Check sheet for the modelled part. Datum: model origin and axes. Units: mm. Face numbers are marked on the shaded views. Give positions to 0.01 mm unless a question says otherwise; leave off trailing zeros. Order: outer loops, then holes, each group sorted by start corner. A loop starts at its lowest first (then second) coordinate and runs counter-clockwise, first axis right, second up.
Item 1: Sectioned sample at D-D on y = -1. Record the boundary of the cut face in (x, z), and give its area (3 significant figures).
Item 2: Release check for a two-part mould opening along Y. For the marked faces 1 and 2 record: released by +Y, released by -Y, zero draft, split by the parting line, or undercut.
Item 3: Material ranges on line 1 along Y through (x, z) = (-6, -0.45); line 2 along X through (y, z) = (-14, 0.75), recorded low to high.
Item 4: Sectioned sample at A-A on x = -5. Record the boundary of the cut face in (y, z), and give its area (3 significant figures).
Item 5: Sectioned sample at C-C on z = 0.6. Record the boundary of the cut face in (x, y), and give its area (3 significant figures).
Item 6: Gauge pin test, flat end, axial feed: P1, Ø9.5, axis at x = -8, y = -2, coming from the +Z side. Record the tip position at first contact, or that the pin passes through.
from build123d import *

# Parameters (mm, degrees)
F0_W     = 12
F0_H     = 12
F1_DEPTH = 1.2
F2_DEPTH = 1.6
F3_R     = 0.4


with BuildPart() as f1:
    # F0 (on Top) → F1 (new body)
    with BuildSketch(Plane.XY):
        with BuildLine():
            Line((12.5, 15.7), (-15, 15.7))
            ThreePointArc((-15, 15.7), (-17.2627416998, 14.7627416998), (-18.2, 12.5))
            Line((-18.2, 12.5), (-18.2, -15))
            ThreePointArc((-18.2, -15), (-17.2627416998, -17.2627416998), (-15, -18.2))
            Line((-15, -18.2), (12.5, -18.2))
            ThreePointArc((12.5, -18.2), (14.7627416998, -17.2627416998), (15.7, -15))
            Line((15.7, -15), (15.7, 12.5))
            ThreePointArc((15.7, 12.5), (14.7627416998, 14.7627416998), (12.5, 15.7))
        make_face()
        with BuildLine():
            ThreePointArc((-17, 12.5), (-16.4142135624, 13.9142135624), (-15, 14.5))
            Line((-15, 14.5), (12.5, 14.5))
            ThreePointArc((12.5, 14.5), (13.9142135624, 13.9142135624), (14.5, 12.5))
            Line((14.5, 12.5), (14.5, -15))
            ThreePointArc((14.5, -15), (13.9142135624, -16.4142135624), (12.5, -17))
            Line((12.5, -17), (-15, -17))
            ThreePointArc((-15, -17), (-16.4142135624, -16.4142135624), (-17, -15))
            Line((-17, -15), (-17, 12.5))
        make_face(mode=Mode.SUBTRACT)
        with BuildLine():
            Line((12.5, 14.5), (-15, 14.5))
            ThreePointArc((-15, 14.5), (-16.4142135624, 13.9142135624), (-17, 12.5))
            Line((-17, 12.5), (-17, -15))
            ThreePointArc((-17, -15), (-16.4142135624, -16.4142135624), (-15, -17))
            Line((-15, -17), (12.5, -17))
            ThreePointArc((12.5, -17), (13.9142135624, -16.4142135624), (14.5, -15))
            Line((14.5, -15), (14.5, 12.5))
            ThreePointArc((14.5, 12.5), (13.9142135624, 13.9142135624), (12.5, 14.5))
        make_face()
        with Locations((-8.5, -8.5)):
            Rectangle(F0_W, F0_H, mode=Mode.SUBTRACT)
        with Locations((6, -8.5)):
            Rectangle(F0_W, F0_H, mode=Mode.SUBTRACT)
        with Locations((-8.5, 6)):
            Rectangle(F0_W, F0_H, mode=Mode.SUBTRACT)
        with Locations((6, 6)):
            Rectangle(F0_W, F0_H, mode=Mode.SUBTRACT)
    extrude(amount=-F1_DEPTH)

    # F0 (on Top) → F2 (join)
    with BuildSketch(Plane.XY):
        with BuildLine():
            Line((12.5, 15.7), (-15, 15.7))
            ThreePointArc((-15, 15.7), (-17.2627416998, 14.7627416998), (-18.2, 12.5))
            Line((-18.2, 12.5), (-18.2, -15))
            ThreePointArc((-18.2, -15), (-17.2627416998, -17.2627416998), (-15, -18.2))
            Line((-15, -18.2), (12.5, -18.2))
            ThreePointArc((12.5, -18.2), (14.7627416998, -17.2627416998), (15.7, -15))
            Line((15.7, -15), (15.7, 12.5))
            ThreePointArc((15.7, 12.5), (14.7627416998, 14.7627416998), (12.5, 15.7))
        make_face()
        with BuildLine():
            ThreePointArc((-17, 12.5), (-16.4142135624, 13.9142135624), (-15, 14.5))
            Line((-15, 14.5), (12.5, 14.5))
            ThreePointArc((12.5, 14.5), (13.9142135624, 13.9142135624), (14.5, 12.5))
            Line((14.5, 12.5), (14.5, -15))
            ThreePointArc((14.5, -15), (13.9142135624, -16.4142135624), (12.5, -17))
            Line((12.5, -17), (-15, -17))
            ThreePointArc((-15, -17), (-16.4142135624, -16.4142135624), (-17, -15))
            Line((-17, -15), (-17, 12.5))
        make_face(mode=Mode.SUBTRACT)
    extrude(amount=F2_DEPTH)

    # F3
    f3_edges = [f1.edges().sort_by_distance(p)[0] for p in [
        (-8.5, -2.5, -1.2),
        (-2.5, -8.5, -1.2),
        (-8.5, -14.5, -1.2),
        (-14.5, -8.5, -1.2),
        (6, -2.5, -1.2),
        (12, -8.5, -1.2),
        (6, -14.5, -1.2),
        (0, -8.5, -1.2),
        (-8.5, 12, -1.2),
        (-2.5, 6, -1.2),
        (-8.5, 0, -1.2),
        (-14.5, 6, -1.2),
        (6, 0, -1.2),
        (0, 6, -1.2),
        (6, 12, -1.2),
        (12, 6, -1.2),
        (-1.25, 15.7, -1.2),
        (-17.262742, 14.762742, -1.2),
        (-18.2, -1.25, -1.2),
        (-17.262742, -17.262742, -1.2),
        (-1.25, -18.2, -1.2),
        (14.762742, -17.262742, -1.2),
        (15.7, -1.25, -1.2),
        (14.762742, 14.762742, -1.2),
    ]]
    fillet(f3_edges, radius=F3_R)


solid = f1.part
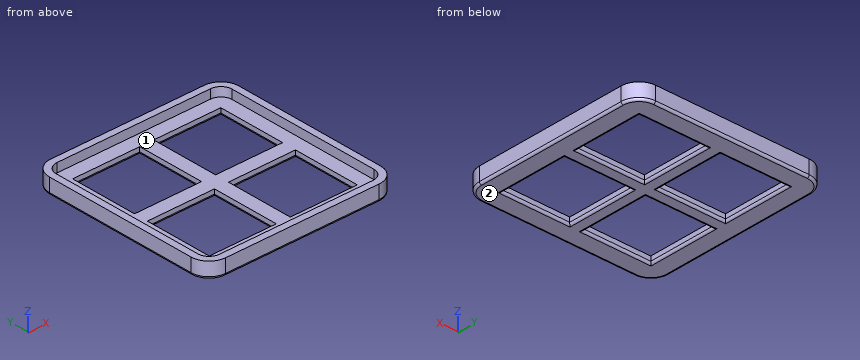
Report:
1. outline: (-18.2, -0.8) arc R0.4 ccw to (-17.8, -1.2) - (15.3, -1.2) arc R0.4 ccw to (15.7, -0.8) - (15.7, 1.6) - (14.5, 1.6) - (14.5, 0) - (-17, 0) - (-17, 1.6) - (-18.2, 1.6) - close
1. area: 44.5 mm2
2. face 1: undercut
2. face 2: zero draft
3. line 1: y = -18.2 to -14.5, -2.5 to 0, 12 to 15.7
3. line 2: x = -18.2 to -17, 14.5 to 15.7
4. outline: (-18.2, -0.8) arc R0.4 ccw to (-17.8, -1.2) - (-14.9, -1.2) arc R0.4 ccw to (-14.5, -0.8) - (-14.5, 0) - (-17, 0) - (-17, 1.6) - (-18.2, 1.6) - close; (-2.5, -0.8) arc R0.4 ccw to (-2.1, -1.2) - (-0.4, -1.2) arc R0.4 ccw to (0, -0.8) - (0, 0) - (-2.5, 0) - close; (12, -0.8) arc R0.4 ccw to (12.4, -1.2) - (15.3, -1.2) arc R0.4 ccw to (15.7, -0.8) - (15.7, 1.6) - (14.5, 1.6) - (14.5, 0) - (12, 0) - close
4. area: 15.5 mm2
5. outline: (-18.2, -15) arc R3.2 ccw to (-15, -18.2) - (12.5, -18.2) arc R3.2 ccw to (15.7, -15) - (15.7, 12.5) arc R3.2 ccw to (12.5, 15.7) - (-15, 15.7) arc R3.2 ccw to (-18.2, 12.5) - close; hole (-17, -15) arc R2 ccw to (-15, -17) - (12.5, -17) arc R2 ccw to (14.5, -15) - (14.5, 12.5) arc R2 ccw to (12.5, 14.5) - (-15, 14.5) arc R2 ccw to (-17, 12.5) - close
5. area: 152 mm2
6. P1: stops at z = 0
